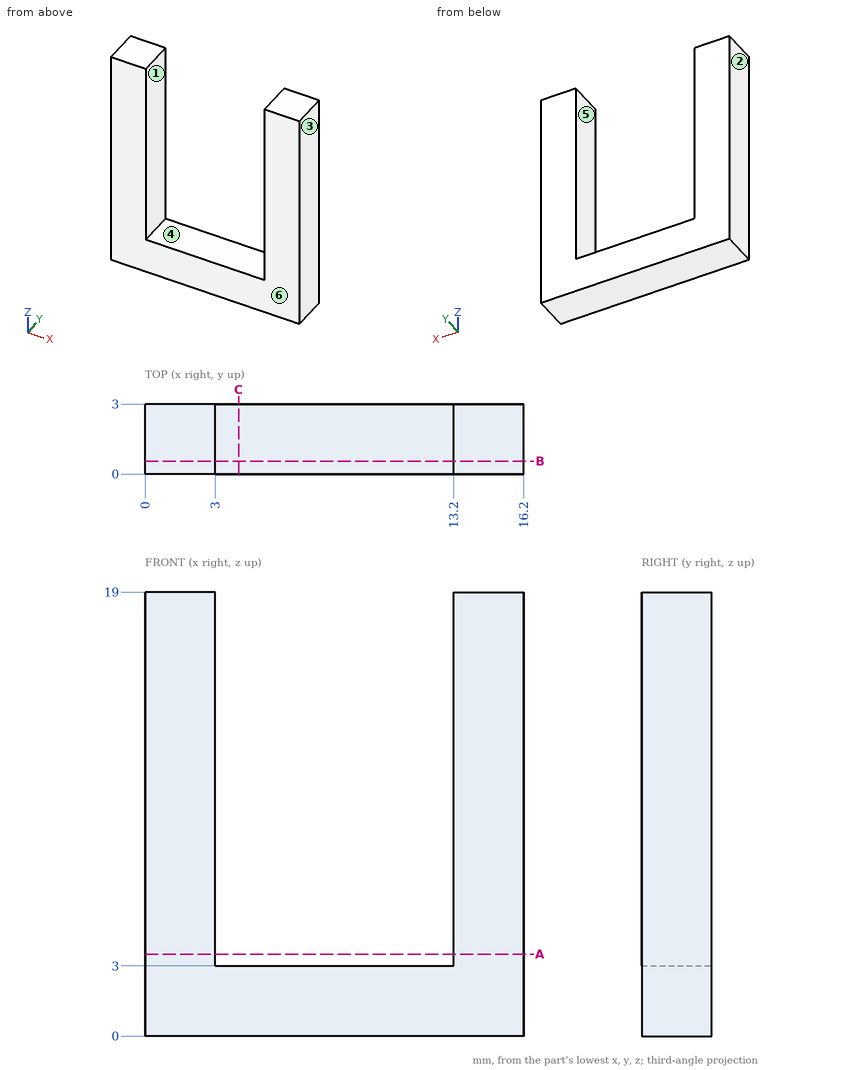
Input: dimensioned drawing with shaded views. Units: mm. Origin: part minimum x, y, z. A direction names the side the tool comes from. Round coordinates to 2 decimals unless told otherwise and drop trailing zeros. Order: outer loops, then holes, each group sorted by start corner. A loop starts at its lowest first (then second) coordinate and runs counter-clockwise, first axis right, second up. Notation, with made-up numbers: (69, -24.5) -> (93, -24.5) arc R29 ccw to (93, 10.5) -> close; hole circle Ø8 at (5.25, 84.25). An arc over 180 degrees is marked (long way). One line per item, written item: value. Start each with the question number.
Q1. Section query B-B (y = 0.55). Return the cut outline in (x, z), plus the area to 3 significant figures.
Q2. Access query for the marked faces 1 and 2. Directions: +Z, -Z, +X, -X, +Y, -Y. A direction counts if a zero-diameter tool reaches every point of the face in a straight line with its end or side. Return the directions, or none.
Q3. Pin query (flat end, axial travel): pin 1 (5 mm diameter, centred on x = 10.5, z = 8, fed in from -Y). Return the tip coordinate at first contact, or that it passes through.
Q4. Section query C-C (x = 4). Return the cut outline in (y, z).
Q5. Draft query along X for the marked faces 3, 4, 5 and 6. Return one class per face: pulls with the +X half, pulls with the -X half, needs draft (parallel to the pull), parting line crosses it, or undercut.
Q6. Section query A-A (z = 3.5). Return the cut outline in (x, y).
Q7. Material intervals for probe 1 along X at (y, z) = (1.35, 6); probe 2 along Z at (x, y) = (12.75, 1), sorted ascending.
Findings below:
1. outline: (0, 0) -> (16.2, 0) -> (16.2, 19) -> (13.2, 19) -> (13.2, 3) -> (3, 3) -> (3, 19) -> (0, 19) -> close
1. area: 145 mm²
2. face 1: +Z, +Y, -Y
2. face 2: +Z, -Z, -X, +Y, -Y
3. pin 1: through
4. outline: (0, 0) -> (3, 0) -> (3, 3) -> (0, 3) -> close
5. face 3: pulls with the +X half
5. face 4: undercut
5. face 5: undercut
5. face 6: needs draft
6. outline: (0, 0) -> (3, 0) -> (3, 3) -> (0, 3) -> close; (13.2, 0) -> (16.2, 0) -> (16.2, 3) -> (13.2, 3) -> close
7. probe 1: 0 to 3, 13.2 to 16.2
7. probe 2: 0 to 3
